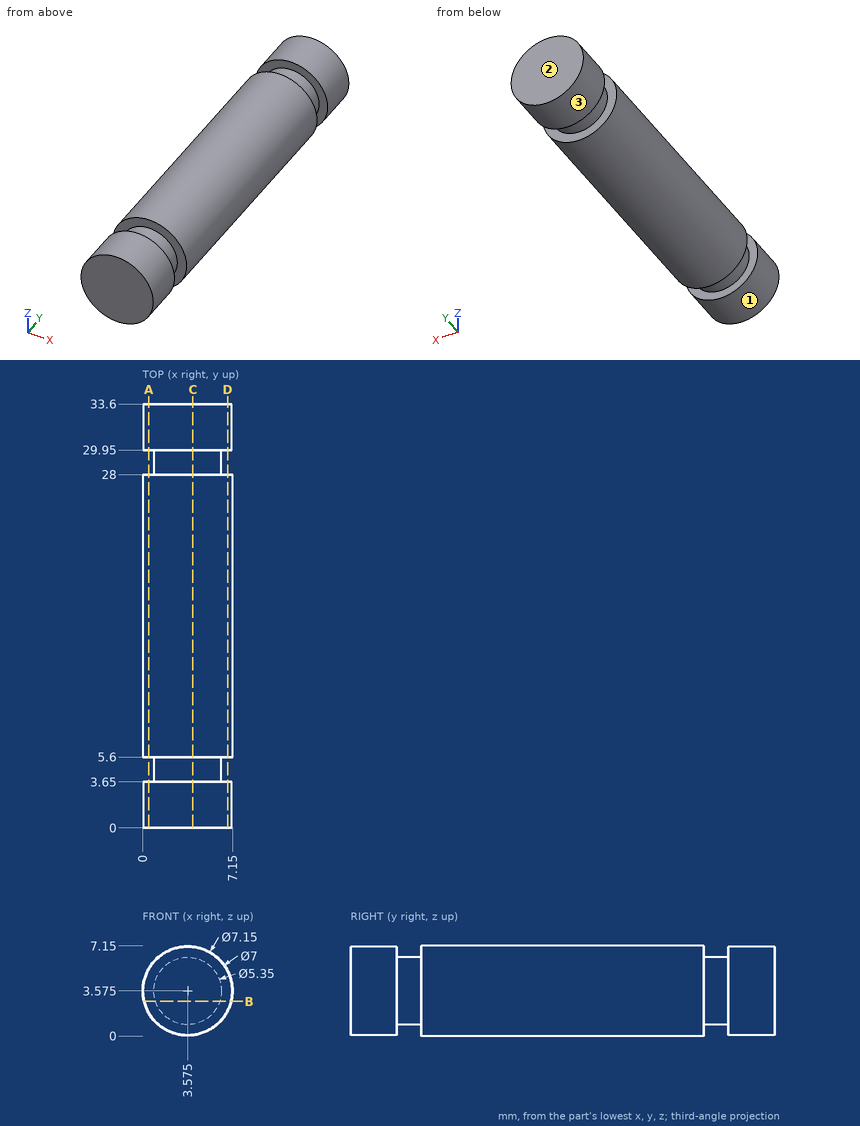
Check sheet for the drawn part. Datum: minimum x, y, z corner. Units: mm. A direction names the side the tool comes from. Coordinates: 2 decimals unless noted, no trailing zeros. Order: outer loops, then holes, each group sorted by start corner. A loop starts at its lowest first (then second) coordinate and runs counter-clockwise, first axis right, second up. Notation, with made-up numbers: (-23.5, 33.25) - (1.5, 33.25) arc R30 ccw to (1.5, 66.25) - close; hole circle Ø3 at (5, 9.25). An arc over 180 degrees is marked (long way). Return JSON: item names as keys, results as strings.
(1) Access from +Z, -Z, +X, -X, +Y, -Y to the whole of each face (thin tool, end or side, straight path). Record for the marked faces 1, 2 and 3.
Filled sheet:
{"face 1": "-Y", "face 2": "+Z, -Z, +X, -X, +Y", "face 3": "+Y"}
(2) Section check A-A, the plane x = 0.5. Record the cut outline in (y, z).
Filled sheet:
{"outline": "(0, 1.9) - (3.65, 1.9) - (3.65, 5.25) - (0, 5.25) - close; (5.6, 1.75) - (28, 1.75) - (28, 5.4) - (5.6, 5.4) - close; (29.95, 1.9) - (33.6, 1.9) - (33.6, 5.25) - (29.95, 5.25) - close"}
(3) Section check C-C, the plane x = 4. Record the cut outline in (y, z), and give its area (3 significant figures).
Filled sheet:
{"outline": "(0, 0.1) - (3.65, 0.1) - (3.65, 0.93) - (5.6, 0.93) - (5.6, 0.03) - (28, 0.03) - (28, 0.93) - (29.95, 0.93) - (29.95, 0.1) - (33.6, 0.1) - (33.6, 7.05) - (29.95, 7.05) - (29.95, 6.22) - (28, 6.22) - (28, 7.12) - (5.6, 7.12) - (5.6, 6.22) - (3.65, 6.22) - (3.65, 7.05) - (0, 7.05) - close", "area": "230 mm^2"}
(4) Section check B-B, the plane z = 2.75. Record the cut outline in (x, y).
Filled sheet:
{"outline": "(0.1, 5.6) - (1.03, 5.6) - (1.03, 3.65) - (0.17, 3.65) - (0.17, 0) - (6.98, 0) - (6.98, 3.65) - (6.12, 3.65) - (6.12, 5.6) - (7.05, 5.6) - (7.05, 28) - (6.12, 28) - (6.12, 29.95) - (6.98, 29.95) - (6.98, 33.6) - (0.17, 33.6) - (0.17, 29.95) - (1.03, 29.95) - (1.03, 28) - (0.1, 28) - close"}
(5) Section check D-D, the plane x = 6.75. Record the cut outline in (y, z).
Filled sheet:
{"outline": "(0, 2.1) - (3.65, 2.1) - (3.65, 5.05) - (0, 5.05) - close; (5.6, 1.93) - (28, 1.93) - (28, 5.22) - (5.6, 5.22) - close; (29.95, 2.1) - (33.6, 2.1) - (33.6, 5.05) - (29.95, 5.05) - close"}
(6) Thickness scan on line 1 along Y through (x, z) = (0.5, 5); line 2 along X through (y, z) = (1, 2.5); line 3 along Z through (x, y) = (3.25, 24). Record the ranges inside material, lowest first.
Filled sheet:
{"line 1": "y = 0 to 3.65, 5.6 to 28, 29.95 to 33.6", "line 2": "x = 0.24 to 6.91", "line 3": "z = 0.01 to 7.14"}
